The listing builds one solid part. Answer for the finished solid, in the listing's coordinates (mm). Face numbers are marked on the shaded views. Give positions to 0.01 mm unless a question says otherwise; leave off trailing zeros. Loops run counter-clockwise (first coordinate to the right, second up) from the corner with the lowest first, then second, coordinate; pieces in that order, holes last.
Item 1: Section C-C, the plane y = 8.5 is taken. Give the vertices of the cut face in (x, z).
Item 2: Section B-B, the plane z = 40 is taken. Give the vertices of the cut face in (x, y).
Item 3: Section D-D, the plane x = -15.5 is taken. Give the vertices of the cut face in (y, z), and give its area (3 significant figures).
Item 4: Section A-A, the plane x = 0 is taken. Give the vertices of the cut face in (y, z).
Item 5: The mould has two halves that part along X. Classify the marked faces 1, 2 and 3: pulls with the +X half, pulls with the -X half, needs draft (parallel to the pull), parting line crosses it, or undercut.
Item 6: Consider line 1 along Z through (x, y) = (5.1, 5); line 2 along X through (y, z) = (8, 40); line 3 along Z through (x, y) = (3.85, 5). Determine where each line is inside the solid, lowest interval first.
Item 7: Each of these flat-tipped pins is pushed along its axis until it touches: pin 1 Ø3 at (y, z) = (4, -44.5) entering from +X; pin 2 Ø1.5 at (y, z) = (2.5, -33.5) entering from -X; pin 3 Ø3 at (x, y) = (-8.5, 5) entering from -Z. Where does it stop, or does it pass through?
from build123d import *

# Parameters (mm, degrees)
SALIENTE_EXTRUIR1_DEPTH  = 10
SALIENTE_EXTRUIR2_START  = -10
SALIENTE_EXTRUIR2_DEPTH  = 10
CROQUIS8_R               = 2
CORTAR_EXTRUIR1_DEPTH    = 10
CROQUIS10_R              = 3.1
CORTAR_EXTRUIR3_DEPTH    = 10
CROQUIS11_W              = 2.5
CROQUIS11_H              = 10
SALIENTE_EXTRUIR5_DEPTH  = 5
CROQUIS13_R              = 2
CORTAR_EXTRUIR4_DEPTH    = 2.5
CROQUIS14_W              = 2.5
CROQUIS14_H              = 10
SALIENTE_EXTRUIR7_DEPTH  = 10
CORTAR_EXTRUIR5_START    = 10
CROQUIS15_R              = 2
CORTAR_EXTRUIR5_DEPTH    = 10
CROQUIS12_R              = 5
CROQUIS12_R_2            = 2
SALIENTE_EXTRUIR8_DEPTH  = 4
SALIENTE_EXTRUIR9_DEPTH  = 1.5
SALIENTE_EXTRUIR10_START = 1
CROQUIS17_W              = 10.235528891
CROQUIS17_H              = 10
CROQUIS17_R              = 2
SALIENTE_EXTRUIR10_DEPTH = 1


with BuildPart() as part:
    # Croquis1 → Saliente-Extruir1 (new body)
    with BuildSketch(Plane(origin=(0, 0, 0), x_dir=(1, 0, 0), z_dir=(0, 1, 0))):
        with BuildLine():
            Line((10, 38.729833462), (10, 32.619012861))
            Line((10, 32.619012861), (10, 31.448370387))
            ThreePointArc((10, 31.448370387), (26.636441204, 19.480759739), (33, 0))
            ThreePointArc((33, 0), (-19.480759739, -26.636441204), (-10, 31.448370387))
            Line((-10, 31.448370387), (-10, 38.729833462))
            ThreePointArc((-10, 38.729833462), (-24.494897428, -31.622776602), (40, 0))
            ThreePointArc((40, 0), (31.622776602, 24.494897428), (10, 38.729833462))
        make_face()
        with BuildLine():
            ThreePointArc((-10, 31.448370387), (-7.522805391, 32.131097072), (-5, 32.619012861))
            Line((-5, 32.619012861), (-5, 39.686269666))
            ThreePointArc((-5, 39.686269666), (-7.515230705, 39.287673734), (-10, 38.729833462))
            Line((-10, 38.729833462), (-10, 31.448370387))
        make_face()
        with BuildLine():
            Line((5, 39.686269666), (5, 32.619012861))
            Line((5, 32.619012861), (10, 32.619012861))
            Line((10, 32.619012861), (10, 38.729833462))
            ThreePointArc((10, 38.729833462), (7.515230705, 39.287673734), (5, 39.686269666))
        make_face()
        with BuildLine():
            Line((10, 39.686269666), (5, 39.686269666))
            ThreePointArc((5, 39.686269666), (7.515230705, 39.287673734), (10, 38.729833462))
            Line((10, 38.729833462), (10, 39.686269666))
        make_face()
        with BuildLine():
            ThreePointArc((-10, 38.729833462), (-7.515230705, 39.287673734), (-5, 39.686269666))
            Line((-5, 39.686269666), (-10, 39.686269666))
            Line((-10, 39.686269666), (-10, 38.729833462))
        make_face()
        with BuildLine():
            Line((10, 32.619012861), (5, 32.619012861))
            ThreePointArc((5, 32.619012861), (7.522805391, 32.131097072), (10, 31.448370387))
            Line((10, 31.448370387), (10, 32.619012861))
        make_face()
        with BuildLine():
            ThreePointArc((-5, 32.619012861), (-3.752728476, 32.785927301), (-2.5, 32.905166768))
            Line((-2.5, 32.905166768), (-2.5, 39.921798557))
            ThreePointArc((-2.5, 39.921798557), (-3.751848673, 39.823656682), (-5, 39.686269666))
            Line((-5, 39.686269666), (-5, 32.619012861))
        make_face()
        with BuildLine():
            ThreePointArc((-5, 39.686269666), (-3.751848673, 39.823656682), (-2.5, 39.921798557))
            Line((-2.5, 39.921798557), (-5, 39.921798557))
            Line((-5, 39.921798557), (-5, 39.686269666))
        make_face()
        with BuildLine():
            Line((2.5, 39.921798557), (2.5, 32.905166768))
            ThreePointArc((2.5, 32.905166768), (3.752728476, 32.785927301), (5, 32.619012861))
            Line((5, 32.619012861), (5, 39.686269666))
            ThreePointArc((5, 39.686269666), (3.751848673, 39.823656682), (2.5, 39.921798557))
        make_face()
        with BuildLine():
            Line((5, 39.921798557), (2.5, 39.921798557))
            ThreePointArc((2.5, 39.921798557), (3.751848673, 39.823656682), (5, 39.686269666))
            Line((5, 39.686269666), (5, 39.921798557))
        make_face()
    extrude(amount=SALIENTE_EXTRUIR1_DEPTH)

    # Croquis2 → Saliente-Extruir2 (add)
    with BuildSketch(Plane(origin=(0, 10, 0), x_dir=(1, 0, 0), z_dir=(0, 1, 0)).offset(SALIENTE_EXTRUIR2_START)):
        with BuildLine():
            ThreePointArc((4.541463415, -45.326829268), (15.280033507, -44.812112406), (19.500878735, -34.924428822))
            ThreePointArc((19.500878735, -34.924428822), (0, -40), (-19.500878735, -34.924428822))
            ThreePointArc((-19.500878735, -34.924428822), (-15.280033507, -44.812112406), (-4.541463415, -45.326829268))
            ThreePointArc((-4.541463415, -45.326829268), (0, -47), (4.541463415, -45.326829268))
        make_face()
    extrude(amount=SALIENTE_EXTRUIR2_DEPTH)

    # Croquis8 → Cortar-Extruir1 (cut)
    with BuildSketch(Plane(origin=(0, 10, 0), x_dir=(1, 0, 0), z_dir=(0, 1, 0))):
        with Locations(Location((9.5, -40, 0), (0, 0, 270))):
            Circle(CROQUIS8_R)
        with Locations(Location((-9.5, -40, 0), (0, 0, 270))):
            Circle(CROQUIS8_R)
    extrude(amount=-CORTAR_EXTRUIR1_DEPTH, mode=Mode.SUBTRACT)

    # Croquis10 → Cortar-Extruir3 (cut)
    with BuildSketch(Plane(origin=(0, 10, 0), x_dir=(1, 0, 0), z_dir=(0, 1, 0))):
        with Locations(Location((0, -40, 0), (0, 0, 270))):
            Circle(CROQUIS10_R)
    extrude(amount=-CORTAR_EXTRUIR3_DEPTH, mode=Mode.SUBTRACT)

    # Croquis11 → Saliente-Extruir5 (add)
    with BuildSketch(Plane(origin=(0, 0, -39.921798557), x_dir=(-1, 0, 0), z_dir=(0, 0, -1))):
        with Locations((3.75, 5)):
            Rectangle(CROQUIS11_W, CROQUIS11_H)
    extrude(amount=SALIENTE_EXTRUIR5_DEPTH)

    # Croquis13 → Cortar-Extruir4 (cut)
    with BuildSketch(Plane(origin=(-2.5, 0, 0), x_dir=(0, 0, -1), z_dir=(1, 0, 0))):
        with Locations((44.921798557, 5)):
            Circle(CROQUIS13_R)
    extrude(amount=-CORTAR_EXTRUIR4_DEPTH, mode=Mode.SUBTRACT)

    # Croquis14 → Saliente-Extruir7 (add)
    with BuildSketch(Plane(origin=(0, 0, -39.921798557), x_dir=(-1, 0, 0), z_dir=(0, 0, -1))):
        with Locations((-3.75, 5)):
            Rectangle(CROQUIS14_W, CROQUIS14_H)
    extrude(amount=SALIENTE_EXTRUIR7_DEPTH)

    # Croquis15 → Cortar-Extruir5 (cut)
    with BuildSketch(Plane(origin=(-2.5, 0, 0), x_dir=(0, 0, -1), z_dir=(1, 0, 0)).offset(CORTAR_EXTRUIR5_START)):
        with Locations(Location((44.921798557, 5, 0), (0, 0, 180))):
            Circle(CROQUIS15_R)
    extrude(amount=-CORTAR_EXTRUIR5_DEPTH, mode=Mode.SUBTRACT)

    # Croquis12 → Saliente-Extruir8 (add)
    with BuildSketch(Plane(origin=(-2.5, 0, 0), x_dir=(0, 0, -1), z_dir=(1, 0, 0))):
        with Locations((44.921798557, 5)):
            Circle(CROQUIS12_R)
        with Locations((44.921798557, 5)):
            Circle(CROQUIS12_R_2, mode=Mode.SUBTRACT)
    extrude(amount=-SALIENTE_EXTRUIR8_DEPTH)

    # Croquis16 → Saliente-Extruir9 (add)
    with BuildSketch(Plane.ZY.offset(5)):
        with BuildLine():
            Line((-44.921798557, 10), (-39.686269666, 10))
            Line((-39.686269666, 10), (-39.686269666, 0))
            Line((-39.686269666, 0), (-44.921798557, 0))
            ThreePointArc((-44.921798557, 0), (-39.921798557, 5), (-44.921798557, 10))
        make_face()
    extrude(amount=SALIENTE_EXTRUIR9_DEPTH)

    # Croquis17 → Saliente-Extruir10 (add)
    with BuildSketch(Plane(origin=(5, 0, 0), x_dir=(0, 0, -1), z_dir=(1, 0, 0)).offset(SALIENTE_EXTRUIR10_START)):
        with Locations((44.804034112, 5)):
            Rectangle(CROQUIS17_W, CROQUIS17_H)
        with Locations((44.921798557, 5)):
            Circle(CROQUIS17_R, mode=Mode.SUBTRACT)
    extrude(amount=-SALIENTE_EXTRUIR10_DEPTH)


solid = part.part
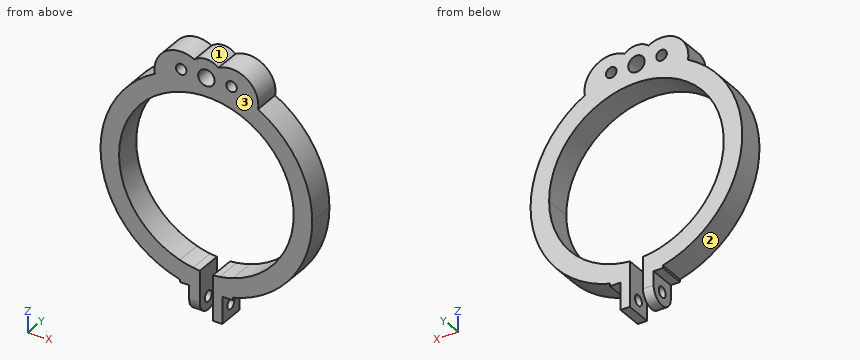
Worked answers:
1. outline: (-19.5, 34.92) arc R40 ccw to (-10, -38.73) - (-10, -39.69) - (-6.5, -39.69) - (-6.5, -48.49) - (-2.5, -48.49) - (-2.5, -32.91) arc R33 cw (long way) to (2.5, -32.91) - (2.5, -49.92) - (6, -49.92) - (6, -39.69) - (10, -39.69) - (10, -38.73) arc R40 ccw to (19.5, 34.92) arc R10.12 ccw to (4.54, 45.33) arc R7 ccw to (-4.54, 45.33) arc R10.12 ccw to start; hole circle Ø4 at (-9.5, 40); hole circle Ø6.2 at (0, 40); hole circle Ø4 at (9.5, 40)
2. outline: (-19, 0) - (-11.5, 0) - (-11.5, 10) - (-19, 10) - close; (-7.5, 0) - (-3.1, 0) - (-3.1, 10) - (-7.5, 10) - close; (3.1, 0) - (7.5, 0) - (7.5, 10) - (3.1, 10) - close; (11.5, 0) - (19, 0) - (19, 10) - (11.5, 10) - close
3. outline: (0, -36.87) - (10, -36.87) - (10, -29.13) - (0, -29.13) - close; (0, 29.13) - (10, 29.13) - (10, 44.65) - (0, 44.65) - close
3. area: 233 mm2
4. outline: (0, 33) - (10, 33) - (10, 36.9) - (0, 36.9) - close; (0, 43.1) - (10, 43.1) - (10, 47) - (0, 47) - close
5. face 1: undercut
5. face 2: pulls with the -X half
5. face 3: needs draft
6. line 1: z = -49.92 to -46.92, -42.92 to -32.6, 32.6 to 45.62
6. line 2: x = -19 to -11.5, -7.5 to -3.1, 3.1 to 7.5, 11.5 to 19
6. line 3: z = -49.92 to -46.92, -42.92 to -32.77, 32.77 to 45.85
7. pin 1: stops at x = 6
7. pin 2: stops at x = -22.97
7. pin 3: stops at z = -39.69
